```python
from build123d import *

# Parameters (mm, degrees)
ESQUISSE1_W             = 42
ESQUISSE1_H             = 46
BOSS_EXTRU_1_DEPTH      = 8
ESQUISSE2_R             = 13.4
ENL_V_MAT_EXTRU_1_DEPTH = 6
ESQUISSE3_R             = 7
ESQUISSE3_R_2           = 1.8
ENL_V_MAT_EXTRU_2_DEPTH = 3
ESQUISSE4_R             = 1.5
ENL_V_MAT_EXTRU_3_DEPTH = 47
ENL_V_MAT_EXTRU_4_REACH = 10
ESQUISSE5_W             = 42
ESQUISSE5_H             = 8


with BuildPart() as part:
    # Esquisse1 → Boss.-Extru.1 (new body)
    with BuildSketch(Plane(origin=(0, 0, 0), x_dir=(1, 0, 0), z_dir=(0, 1, 0))):
        with Locations((21, 23)):
            Rectangle(ESQUISSE1_W, ESQUISSE1_H)
    extrude(amount=BOSS_EXTRU_1_DEPTH)

    # Esquisse2 → Enlèv. mat.-Extru.1 (cut)
    with BuildSketch(Plane(origin=(0, 8, 0), x_dir=(1, 0, 0), z_dir=(0, 1, 0))):
        with Locations((21, 23)):
            Circle(ESQUISSE2_R)
    extrude(amount=-ENL_V_MAT_EXTRU_1_DEPTH, mode=Mode.SUBTRACT)

    # Esquisse3 → Enlèv. mat.-Extru.2 (cut, through all)
    with BuildSketch(Plane(origin=(0, 2, 0), x_dir=(1, 0, 0), z_dir=(0, 1, 0))):
        with Locations((21, 23)):
            Circle(ESQUISSE3_R)
        with Locations((21, 33)):
            Circle(ESQUISSE3_R_2)
        with Locations((31, 23)):
            Circle(ESQUISSE3_R_2)
        with Locations((21, 13)):
            Circle(ESQUISSE3_R_2)
        with Locations((11, 23)):
            Circle(ESQUISSE3_R_2)
    extrude(amount=-ENL_V_MAT_EXTRU_2_DEPTH, mode=Mode.SUBTRACT)

    # Esquisse4 → Enlèv. mat.-Extru.3 (cut, through all)
    with BuildSketch(Plane(origin=(0, 0, -46), x_dir=(-1, 0, 0), z_dir=(0, 0, -1))):
        with Locations((-38, 4)):
            Circle(ESQUISSE4_R)
        with Locations((-4, 4)):
            Circle(ESQUISSE4_R)
    extrude(amount=-ENL_V_MAT_EXTRU_3_DEPTH, mode=Mode.SUBTRACT)

    # Esquisse5 → Enlèv. mat.-Extru.4 (cut, up to next)
    with BuildSketch(Plane(origin=(0, 8, 0), x_dir=(1, 0, 0), z_dir=(0, 1, 0)), mode=Mode.PRIVATE) as enl_v_mat_extru_4_sk1:
        with Locations((21, 42)):
            Rectangle(ESQUISSE5_W, ESQUISSE5_H)
    enl_v_mat_extru_4_tool1 = extrude(enl_v_mat_extru_4_sk1.sketch, amount=-ENL_V_MAT_EXTRU_4_REACH, mode=Mode.PRIVATE) & part.part
    add(enl_v_mat_extru_4_tool1.solids().sort_by_distance((21, 8, -42))[0], mode=Mode.SUBTRACT)


solid = part.part
```
Source: CAD feature listing. Evaluate the final solid. Frame: model axes, mm. A direction names the side the tool comes from. Give positions to 0.01 mm unless a question says otherwise; leave off trailing zeros. Loops run counter-clockwise (first coordinate to the right, second up) from the corner with the lowest first, then second, coordinate; pieces in that order, holes last. Notation, with made-up numbers: (-17, -7) -> (1, -7) arc R14 ccw to (1, 10) -> close; hole circle Ø3 at (31, 85.25). An arc over 180 degrees is marked (long way). Put each result on its own line as item: value. Start each with the question number.
1) Material intervals for probe 1 along X at (y, z) = (1, -23); probe 2 along Z at (x, y) = (21, 1); probe 3 along Z at (x, y) = (11, 1), sorted ascending.
2) Cut plane B-B (z = -23). Return loops of the section in (x, y).
3) Cut plane D-D (y = 3.25). Return loops of the section in (x, z).
4) Reachability of faces 1 (the face through (33.781, 5.042, -27.025)), 2 (the face through (22.717, 1.014, -13.541)) from +Z, -Z, +X, -X, +Y, -Y: full face, straight path, thin tool, end or side. Return the list, or none.
5) Contact query for a flat-ended pin moving along its axis: P1, Ø6, axis at x = 15.5, z = -28, coming from the +Y side. Output: stop coordinate, or through.
6) Draft query along X for faces 3 (the face through (0, 4, -19)), 4 (the face through (20.766, 1.014, -34.785)), 5 (the face through (21, 4, 0)). Return one class per face: released by +X, released by -X, zero draft, split by the parting line, or undercut.
7) Cut plane C-C (x = 4). Return loops of the section in (y, z).
8) Cut plane A-A (x = 21). Return loops of the section in (y, z), then the cut area to 3 significant figures.
Results are:
1. probe 1: x = 0 to 9.2, 12.8 to 14, 28 to 29.2, 32.8 to 42
1. probe 2: z = -38 to -34.8, -31.2 to -30, -16 to -14.8, -11.2 to 0
1. probe 3: z = -38 to -24.8, -21.2 to 0
2. outline: (0, 0) -> (9.2, 0) -> (9.2, 2) -> (7.6, 2) -> (7.6, 8) -> (0, 8) -> close; (12.8, 0) -> (14, 0) -> (14, 2) -> (12.8, 2) -> close; (28, 0) -> (29.2, 0) -> (29.2, 2) -> (28, 2) -> close; (32.8, 0) -> (42, 0) -> (42, 8) -> (34.4, 8) -> (34.4, 2) -> (32.8, 2) -> close; hole circle Ø3 at (4, 4); hole circle Ø3 at (38, 4)
3. outline: (0, -38) -> (2.7, -38) -> (2.7, 0) -> (0, 0) -> close; (5.3, -38) -> (36.7, -38) -> (36.7, 0) -> (5.3, 0) -> close; (39.3, -38) -> (42, -38) -> (42, 0) -> (39.3, 0) -> close; hole circle Ø26.8 at (21, -23)
4. face 1: +Y
4. face 2: +Y, -Y
5. P1: stops at y = 2
6. face 3: released by -X
6. face 4: undercut
6. face 5: zero draft
7. outline: (0, -38) -> (2.5, -38) -> (2.5, 0) -> (0, 0) -> close; (5.5, -38) -> (8, -38) -> (8, 0) -> (5.5, 0) -> close
8. outline: (0, -38) -> (8, -38) -> (8, -36.4) -> (2, -36.4) -> (2, -34.8) -> (0, -34.8) -> close; (0, -31.2) -> (2, -31.2) -> (2, -30) -> (0, -30) -> close; (0, -16) -> (2, -16) -> (2, -14.8) -> (0, -14.8) -> close; (0, -11.2) -> (2, -11.2) -> (2, -9.6) -> (8, -9.6) -> (8, 0) -> (0, 0) -> close
8. area: 101 mm2
